Verification items for the finished model (mm, model axes). Face numbers are marked on the shaded views. A direction names the side the tool comes from. Round coordinates to 2 decimals unless told otherwise and drop trailing zeros. Order: outer loops, then holes, each group sorted by start corner. A loop starts at its lowest first (then second) coordinate and runs counter-clockwise, first axis right, second up. Notation, with made-up numbers: M -1,88.25 L 5,88.25 A4 ccw 5,94.25 Z; hole C 72,-32.5 d6. An arc over 180 degrees is marked long. Use CSV: the item, a comma, the result in double quotes. Start each with the question number.
Q1. Sectioned sample at A-A (z = -5.75). Enter the section's corners in (x, y) (1 decimal), and give its area (3 significant figures).
Q2. Scan lines: line 1 (X direction, y = 10.5, z = 3.5) (3 decimals); line 2 (X direction, y = 24, z = -0.5); line 3 (Z direction, x = 30.5, y = 14) (3 decimals). Record each from-to range of solid material in increasing order.
Q3. Sectioned sample at B-B (y = 10). Enter the section's corners in (x, z) (1 decimal).
Q4. Sectioned sample at C-C (x = 254). Enter the section's corners in (y, z) (1 decimal), and give its area (3 significant figures).
Q5. Set-up check for the marked faces 1 and 2: record each of +Z, -Z, +X, -X, +Y, -Y from which the full face is reachable in a straight line by a thin tool's end or side.
Q6. Gauge pin test, flat ends, axial feed: pin 1 Ø8.5 at (y, z) = (22.5, 3) entering from +X; pin 2 Ø4 at (y, z) = (25, -8.5) entering from -X; pin 3 Ø1 at (x, z) = (-1.5, -1) entering from +Y. Record the tip position at first contact, or that the pin passes through.
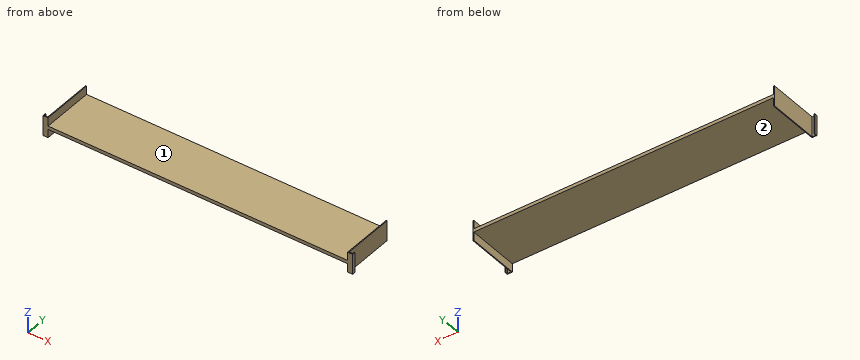
```python
from build123d import *

# Parameters (mm, degrees)
SKETCH1_W           = 282.575
SKETCH1_H           = 3.175
SKETCH1_W_2         = 4.7625
SKETCH1_H_2         = 19.05
BOSS_EXTRUDE1_DEPTH = 49.2125
CUT_EXTRUDE1_DEPTH  = 293.143135402


with BuildPart() as part:
    # Sketch1 → Boss-Extrude1 (new body)
    with BuildSketch(Plane(origin=(0, 0, 0), x_dir=(1, 0, 0), z_dir=(0, 1, 0))):
        with Locations((141.2875, 1.5875)):
            Rectangle(SKETCH1_W, SKETCH1_H)
        with Locations((-2.38125, 1.5875)):
            Rectangle(SKETCH1_W_2, SKETCH1_H_2)
        with Locations((284.95625, 1.5875)):
            Rectangle(SKETCH1_W_2, SKETCH1_H_2)
    extrude(amount=BOSS_EXTRUDE1_DEPTH)

    # Sketch2 → Cut-Extrude1 (cut, through all)
    with BuildSketch(Plane.XY.offset(7.9375)):
        Polygon((-4.7625, 2.81851333), (-3.96875, 2.81851333), (-3.96875, 0.79375), (-0.79375, 0.79375), (-0.79375, 49.2125), (-4.7625, 49.2125), align=None)
        Polygon((287.3375, 2.81851333), (286.54375, 2.81851333), (286.54375, 0.79375), (283.36875, 0.79375), (283.36875, 49.2125), (287.3375, 49.2125), align=None)
    extrude(amount=-CUT_EXTRUDE1_DEPTH, mode=Mode.SUBTRACT)


solid = part.part
```
Verdict:
1,outline,"M -4.8,0 L 0,0 L 0,49.2 L -0.8,49.2 L -0.8,0.8 L -4,0.8 L -4,2.8 L -4.8,2.8 Z; M 282.6,0 L 287.3,0 L 287.3,2.8 L 286.5,2.8 L 286.5,0.8 L 283.4,0.8 L 283.4,49.2 L 282.6,49.2 Z"
1,area,"87.6 mm²"
2,line 1,"x = -0.794 to 0, 282.575 to 283.369"
2,line 2,"x = -0.79 to 283.37"
2,line 3,"z = -3.175 to 0"
3,outline,"M -0.8,-11.1 L 0,-11.1 L 0,-3.2 L 282.6,-3.2 L 282.6,-11.1 L 283.4,-11.1 L 283.4,7.9 L 282.6,7.9 L 282.6,0 L 0,0 L 0,7.9 L -0.8,7.9 Z"
4,outline,"M 0,-3.2 L 49.2,-3.2 L 49.2,0 L 0,0 Z"
4,area,"156 mm²"
5,face 1,"+Z, +Y, -Y"
5,face 2,"-Z, +Y, -Y"
6,pin 1,"stops at x = 283.37"
6,pin 2,"stops at x = -0.79"
6,pin 3,"stops at y = 0.79"
